Geometry: final body of the model. Coordinates: model frame, mm. A direction names the side the tool comes from. Give positions to 0.01 mm unless a question says otherwise; leave off trailing zeros. Loops run counter-clockwise (first coordinate to the right, second up) from the corner with the lowest first, then second, coordinate; pieces in that order, holes last. Notation, with made-up numbers: (33.25, -33) - (67.25, -33) arc R14 ccw to (67.25, -11) - close; hole circle Ø4 at (3.5, -4). An arc over 180 degrees is marked (long way). Answer in a Markdown table with one row per item.
from build123d import *

# Parameters (mm, degrees)
SKETCH1_W           = 50.8
SKETCH1_H           = 5.08
BOSS_EXTRUDE1_DEPTH = 7.62
SKETCH2_R           = 1.778
BOSS_EXTRUDE2_DEPTH = 5.08
BOSS_EXTRUDE3_START = 5.08
SKETCH3_R           = 1.778
BOSS_EXTRUDE3_DEPTH = 5.08
SKETCH4_W           = 2.032
SKETCH4_H           = 5.08
BOSS_EXTRUDE4_DEPTH = 2.54
BOSS_EXTRUDE5_DEPTH = 1.27
SKETCH6_W           = 2.032
SKETCH6_H           = 5.08
BOSS_EXTRUDE6_DEPTH = 2.54
BOSS_EXTRUDE7_START = -1.27
BOSS_EXTRUDE7_DEPTH = 1.27
SKETCH8_R           = 1.778
CUT_EXTRUDE1_DEPTH  = 61.588451045


with BuildPart() as part:
    # Sketch1 → Boss-Extrude1 (new body)
    with BuildSketch(Plane.XY):
        with Locations((25.4, -2.54)):
            Rectangle(SKETCH1_W, SKETCH1_H)
    extrude(amount=BOSS_EXTRUDE1_DEPTH)

    # Sketch2 → Boss-Extrude2 (add)
    with BuildSketch(Plane.XY.offset(7.62)):
        with Locations((2.54, -2.54)):
            Circle(SKETCH2_R)
    extrude(amount=BOSS_EXTRUDE2_DEPTH)

    # Sketch3 → Boss-Extrude3 (add)
    with BuildSketch(Plane(origin=(0, 0, 0), x_dir=(-1, 0, 0), z_dir=(0, 0, -1)).offset(BOSS_EXTRUDE3_START)):
        with Locations(Location((-2.54, -2.54, 0), (0, 0, 180))):
            Circle(SKETCH3_R)
    extrude(amount=-BOSS_EXTRUDE3_DEPTH)

    # Sketch4 → Boss-Extrude4 (add)
    with BuildSketch(Plane.XY.offset(7.62)):
        with Locations((49.784, -2.54)):
            Rectangle(SKETCH4_W, SKETCH4_H)
    extrude(amount=BOSS_EXTRUDE4_DEPTH)

    # Sketch5 → Boss-Extrude5 (add)
    with BuildSketch(Plane.XY.offset(10.16)):
        with BuildLine():
            Line((50.8, 0), (55.88, 0))
            ThreePointArc((55.88, 0), (58.42, -2.54), (55.88, -5.08))
            Line((55.88, -5.08), (50.8, -5.08))
            Line((50.8, -5.08), (50.8, 0))
        make_face()
    extrude(amount=-BOSS_EXTRUDE5_DEPTH)

    # Sketch6 → Boss-Extrude6 (add)
    with BuildSketch(Plane(origin=(0, 0, 0), x_dir=(-1, 0, 0), z_dir=(0, 0, -1))):
        with Locations((-49.784, -2.54)):
            Rectangle(SKETCH6_W, SKETCH6_H)
    extrude(amount=BOSS_EXTRUDE6_DEPTH)

    # Sketch7 → Boss-Extrude7 (add)
    with BuildSketch(Plane(origin=(0, 0, -2.54), x_dir=(-1, 0, 0), z_dir=(0, 0, -1)).offset(BOSS_EXTRUDE7_START)):
        with BuildLine():
            Line((-48.768, 0), (-55.88, 0))
            ThreePointArc((-55.88, 0), (-58.42, -2.54), (-55.88, -5.08))
            Line((-55.88, -5.08), (-48.768, -5.08))
            Line((-48.768, -5.08), (-48.768, 0))
        make_face()
    extrude(amount=BOSS_EXTRUDE7_DEPTH)

    # Sketch8 → Cut-Extrude1 (cut, through all)
    with BuildSketch(Plane(origin=(0, 0, -2.54), x_dir=(-1, 0, 0), z_dir=(0, 0, -1))):
        with Locations((-55.88, -2.54)):
            Circle(SKETCH8_R)
    extrude(amount=-CUT_EXTRUDE1_DEPTH, mode=Mode.SUBTRACT)


solid = part.part
Q1. Cut plane D-D (z = 2). Output: boundary loops of the cut face in (x, y), and give its area (3 significant figures).
Check values:
| item | result |
|---|---|
| outline | (0, -5.08) - (50.8, -5.08) - (50.8, 0) - (0, 0) - close |
| area | 258 mm² |
Q2. Reachability of faces 1 (the cylindrical face through (1.1, -1.5, -2.6)), 2 (the flat face through (48.768, -3, -1)), 3 (the flat face through (48.768, -3, 9)), 4 (the flat face through (53, -3, -2.54)), 5 (the flat face through (50.8, -3, 4)) from +Z, -Z, +X, -X, +Y, -Y: full face, straight path, thin tool, end or side. Return the list, or none.
Check values:
| item | result |
|---|---|
| face 1 | -Z |
| face 2 | -Z, +Y, -Y |
| face 3 | +Z, +Y, -Y |
| face 4 | -Z, +X, +Y, -Y |
| face 5 | +X, +Y, -Y |
Q3. Cut plane C-C (x = 2.54). Output: boundary loops of the cut face in (y, z), and give its area (3 significant figures).
Check values:
| item | result |
|---|---|
| outline | (-5.08, 0) - (-4.32, 0) - (-4.32, -5.08) - (-0.76, -5.08) - (-0.76, 0) - (0, 0) - (0, 7.62) - (-0.76, 7.62) - (-0.76, 12.7) - (-4.32, 12.7) - (-4.32, 7.62) - (-5.08, 7.62) - close |
| area | 74.8 mm² |
Q4. Cut plane B-B (z = 9.5). Output: boundary loops of the cut face in (x, y).
Check values:
| item | result |
|---|---|
| outline | circle Ø3.56 at (2.54, -2.54); (48.77, -5.08) - (55.88, -5.08) arc R2.54 ccw to (55.88, 0) - (48.77, 0) - close; hole circle Ø3.56 at (55.88, -2.54) |
Q5. Draft query along Y for faces 6 (the cylindrical face through (1.13, -3.62, 10.12)), 7 (the cylindrical face through (57.656, -2.462, 9.516)), 8 (the flat face through (53, -3, 10.16)). Return one class per face: pulls with the +Y half, pulls with the -Y half, needs draft (parallel to the pull), parting line crosses it, or undercut.
Check values:
| item | result |
|---|---|
| face 6 | parting line crosses it |
| face 7 | undercut |
| face 8 | needs draft |
Q6. Material intervals for line 1 along Y through (x, z) = (55.88, 9.75); line 2 along X through (y, z) = (-3.2, 1); line 3 along Z through (x, y) = (28.5, -0.45), sorted ascending.
Check values:
| item | result |
|---|---|
| line 1 | -5.08 to -4.32, -0.76 to 0 |
| line 2 | 0 to 50.8 |
| line 3 | 0 to 7.62 |
Q7. Cut plane A-A (y = -2.54). Output: boundary loops of the cut face in (x, z), and give its area (3 significant figures).
Check values:
| item | result |
|---|---|
| outline | (0, 0) - (0.76, 0) - (0.76, -5.08) - (4.32, -5.08) - (4.32, 0) - (48.77, 0) - (48.77, -2.54) - (54.1, -2.54) - (54.1, -1.27) - (50.8, -1.27) - (50.8, 8.89) - (54.1, 8.89) - (54.1, 10.16) - (48.77, 10.16) - (48.77, 7.62) - (4.32, 7.62) - (4.32, 12.7) - (0.76, 12.7) - (0.76, 7.62) - (0, 7.62) - close; (57.66, -2.54) - (58.42, -2.54) - (58.42, -1.27) - (57.66, -1.27) - close; (57.66, 8.89) - (58.42, 8.89) - (58.42, 10.16) - (57.66, 10.16) - close |
| area | 444 mm² |
Q8. First-contact query: pin 1 (1.5 mm diameter, centred on x = 24, y = -2.5, fed in from -Z); pin 2 (2 mm diameter, centred on y = -3, z = -1.5, fed in from -X); pin 3 (1.5 mm diameter, centred on x = 16, z = -1, fed in from +Y). Flat tips, straight axial feed; report the tip coordinate or a pass-through.
Check values:
| item | result |
|---|---|
| pin 1 | z = 0 |
| pin 2 | x = 0.76 |
| pin 3 | through |
